The drawing under review shows one solid part. Ordinate dimensions are in mm from its lowest x, y, z. A direction names the side the tool comes from. Coordinates: 2 decimals unless noted, no trailing zeros.
1) Machinability: for the marked faces 4 and 5, which of the approach directions +Z, -Z, +X, -X, +Y, -Y give a long, thin tool a straight path to every point of the face, cutting with its end or side? Answer none if there is none.
2) For line 1 (Y direction, x = 53.5, z = 16.5) (1 decimal); line 2 (X direction, y = 42.5, z = 50.5) (1 decimal); line 3 (X direction, y = 66.5, z = 89.5) (1 decimal), list the stretches that pass through material, from the lowest coordinate up.
3) Mouldability with a two-part tool opening along Y and no side actions: class the marked faces 1, 2 and 3 as released by +Y, released by -Y, zero draft, split by the parting line, or undercut.
4) For P1, Ø1, axis at y = 85, z = 38, coming from the -X side; P2, Ø6, axis at x = 46.5, z = 88.5, coming from the -Y side; P3, Ø12, axis at x = 66.5, z = 26.5, coming from the -Y side, all flat-tipped, find the tip position at first contact; note any pin that passes through.
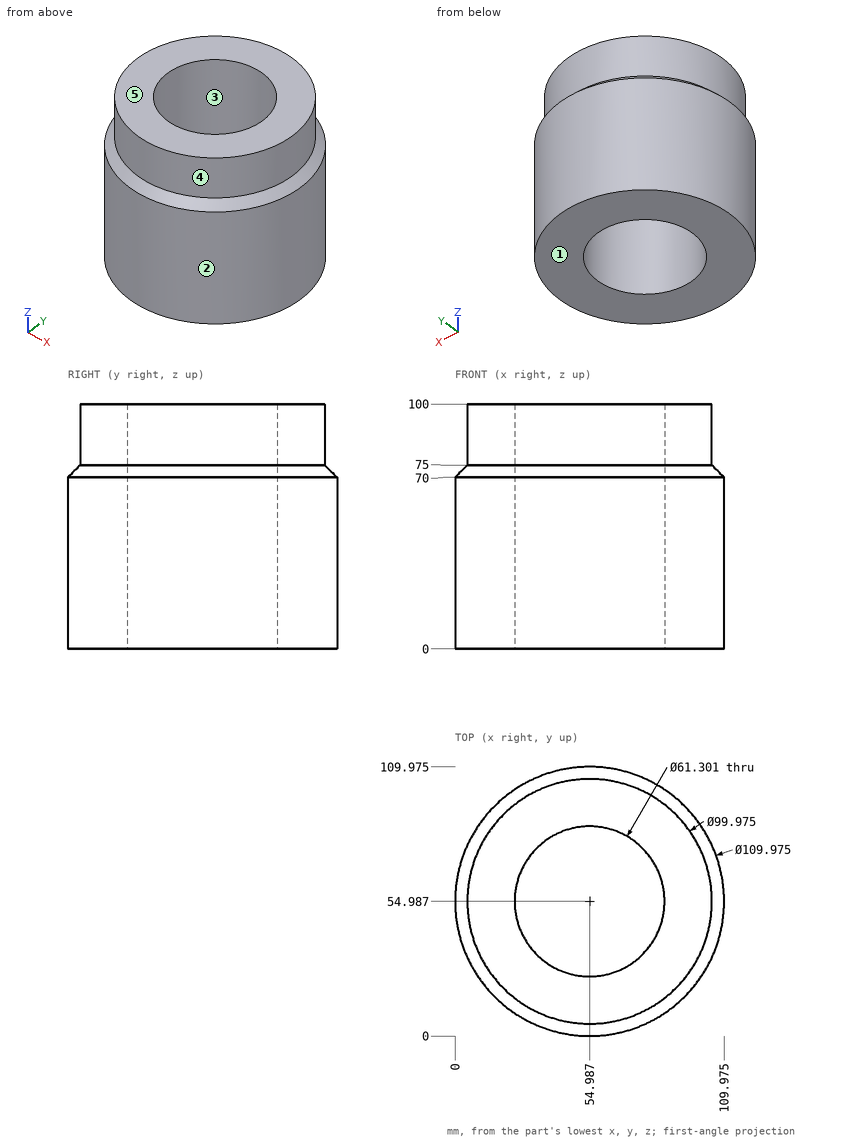
Geometry results:
1. face 4: +Z
1. face 5: +Z, +X, -X, +Y, -Y
2. line 1: y = 0 to 24.4, 85.6 to 110
2. line 2: x = 1.4 to 27, 83 to 108.5
2. line 3: x = 6.3 to 26.6, 83.4 to 103.6
3. face 1: zero draft
3. face 2: split by the parting line
3. face 3: undercut
4. P1: stops at x = 8.59
4. P2: stops at y = 5.3
4. P3: stops at y = 0.28
